The model under review builds one solid part; all positions refer to its coordinate system, in mm. A direction names the side the tool comes from. Round coordinates to 2 decimals unless told otherwise and drop trailing zeros. Loops run counter-clockwise (first coordinate to the right, second up) from the corner with the lowest first, then second, coordinate; pieces in that order, holes last. Notation, with made-up numbers: (11, -36.5) - (49, -36.5) arc R21 ccw to (49, -9.5) - close; hole circle Ø11 at (-36.5, -22.5). An arc over 180 degrees is marked (long way). Answer as CSV lines item,"result".
from build123d import *

# Parameters (mm, degrees)
IZIM1_R                     = 2.2
Y_KSEKLIK_EKSTR_ZYON1_DEPTH = 20
IZIM2_R                     = 5.35
IZIM2_R_2                   = 2.2
Y_KSEKLIK_EKSTR_ZYON2_DEPTH = 12
KES_EKSTR_ZYON1_DEPTH       = 10


with BuildPart() as part:
    # Çizim1 → Yükseklik-Ekstrüzyon1 (new body)
    with BuildSketch(Plane(origin=(0, 0, 0), x_dir=(1, 0, 0), z_dir=(0, 1, 0))):
        with BuildLine():
            Line((-4.527692569, 2.85), (4.527692569, 2.85))
            ThreePointArc((4.527692569, 2.85), (0, -5.35), (-4.527692569, 2.85))
        make_face()
        with Locations(Location((0, 0, 0), (0, 0, 270))):
            Circle(IZIM1_R, mode=Mode.SUBTRACT)
    extrude(amount=Y_KSEKLIK_EKSTR_ZYON1_DEPTH)

    # Çizim2 → Yükseklik-Ekstrüzyon2 (add)
    with BuildSketch(Plane(origin=(0, 20, 0), x_dir=(1, 0, 0), z_dir=(0, 1, 0))):
        with Locations(Location((0, 0, 0), (0, 0, 32.188761118))):
            Circle(IZIM2_R)
        with Locations(Location((0, 0, 0), (0, 0, 270))):
            Circle(IZIM2_R_2, mode=Mode.SUBTRACT)
    extrude(amount=Y_KSEKLIK_EKSTR_ZYON2_DEPTH)

    # Çizim3 → Kes-Ekstrüzyon1 (cut)
    with BuildSketch(Plane(origin=(0, 32, 0), x_dir=(1, 0, 0), z_dir=(0, 1, 0))):
        with BuildLine():
            Line((-1.673320053, 2.55), (1.673320053, 2.55))
            ThreePointArc((1.673320053, 2.55), (0, -3.05), (-1.673320053, 2.55))
        make_face()
    extrude(amount=-KES_EKSTR_ZYON1_DEPTH, mode=Mode.SUBTRACT)


solid = part.part
1. Take a section at D-D (z = 2.75). State the section outline as (x, y) points, plus the area to 3 significant figures.
Numbers:
outline,"(-4.59, 0) - (4.59, 0) - (4.59, 32) - (1.32, 32) - (1.32, 22) - (-1.32, 22) - (-1.32, 32) - (-4.59, 32) - close"
area,"267 mm²"
2. Draft analysis for pull direction X (two halves, no side actions). For faces 4 (the face through (-1.1, 0, 2.1)), 5 (the face through (-1.3, 22, 2.1)), state which applies: +X half, -X half, draft (parallel to the pull), parting line (faces both ways), or undercut.
Numbers:
face 4,"draft"
face 5,"undercut"
3. Take a section at B-B (x = 0). State the section outline as (y, z) points, plus the area to 3 significant figures.
Numbers:
outline,"(0, -2.85) - (20, -2.85) - (20, -5.35) - (32, -5.35) - (32, -2.55) - (22, -2.55) - (22, -2.2) - (0, -2.2) - close; (0, 2.2) - (22, 2.2) - (22, 3.05) - (32, 3.05) - (32, 5.35) - (0, 5.35) - close"
area,"140 mm²"
4. Wall thickness on probe 1 along X at (y, z) = (26.5, 0); probe 2 along Z at (x, y) = (0, 12); probe 3 along X at (y, z) = (12.5, 0): over which ranges is each line inside the solid? List them lowest first.
Numbers:
probe 1,"x = -5.35 to -3.05, 3.05 to 5.35"
probe 2,"z = -2.85 to -2.2, 2.2 to 5.35"
probe 3,"x = -5.35 to -2.2, 2.2 to 5.35"
5. Clearance check with flat-ended pins moving along their axes: pin 1 (2 mm diameter, centred on x = 1.5, z = -4, fed in from -Y); pin 2 (3.5 mm diameter, centred on x = 0, z = 0, fed in from +Y); pin 3 (2 mm diameter, centred on x = 3.5, y = 25, fed in from +Z); pin 4 (1 mm diameter, centred on x = -4, y = 22.5, fed in from -Z). State where each tip first meets the part, or that it passes through.
Numbers:
pin 1,"stops at y = 20"
pin 2,"passes through"
pin 3,"stops at z = 4.73"
pin 4,"stops at z = -4.05"
6. Take a section at A-A (z = 0). State the section outline as (x, y) points.
Numbers:
outline,"(-5.35, 0) - (-2.2, 0) - (-2.2, 22) - (-3.05, 22) - (-3.05, 32) - (-5.35, 32) - close; (2.2, 0) - (5.35, 0) - (5.35, 32) - (3.05, 32) - (3.05, 22) - (2.2, 22) - close"
7. Tool access review of faces 1 (the face through (0, 32, -3)), 2 (the face through (0.11, 27.07, 3.05)), 3 (the face through (0, 20, -4)): name each direction out of +Z, -Z, +X, -X, +Y, -Y from which nothing blocks a thin tool from reaching the whole face with its end or side.
Numbers:
face 1,"+Z, -Z, +X, -X, +Y"
face 2,"+Y"
face 3,"-Z, +X, -X, -Y"
8. Take a section at C-C (y = 16.5). State the section outline as (x, z) points.
Numbers:
outline,"(-4.53, -2.85) - (4.53, -2.85) arc R5.35 ccw (long way) to start; hole circle Ø4.4 at (0, 0)"
